from build123d import *

# Parameters (mm, degrees)
CROQUIS1_R              = 2.034348523
CROQUIS1_R_2            = 3
SALIENTE_EXTRUIR1_DEPTH = 3
SALIENTE_EXTRUIR2_DEPTH = 3
MATRIZC1_COUNT          = 8
MATRIZC1_ANGLE          = 128
CROQUIS4_R              = 1.53
CORTAR_EXTRUIR1_DEPTH   = 10


with BuildPart() as part:
    # Croquis1 → Saliente-Extruir1 (new body)
    with BuildSketch(Plane(origin=(0, 0, 0), x_dir=(1, 0, 0), z_dir=(0, 1, 0))):
        with BuildLine():
            Line((-5, -10.339498295), (-5, -30))
            ThreePointArc((-5, -30), (0, -35), (5, -30))
            Line((5, -30), (5, -10.339498295))
            ThreePointArc((5, -10.339498295), (0, 11.485), (-5, -10.339498295))
        make_face()
        with Locations((0, -30)):
            Circle(CROQUIS1_R, mode=Mode.SUBTRACT)
        Circle(CROQUIS1_R_2, mode=Mode.SUBTRACT)
    extrude(amount=SALIENTE_EXTRUIR1_DEPTH)

    # Croquis3 → Saliente-Extruir2 (add)
    with BuildSketch(Plane(origin=(0, 0, 0), x_dir=(1, 0, 0), z_dir=(0, 1, 0))):
        with BuildLine():
            Line((-1.1484375, 12.965487086), (-1.1484375, 11.427436996))
            ThreePointArc((-1.1484375, 11.427436996), (0, 11.485), (1.1484375, 11.427436996))
            Line((1.1484375, 11.427436996), (1.1484375, 12.965487086))
            Line((1.1484375, 12.965487086), (0.57421875, 14.536162804))
            ThreePointArc((0.57421875, 14.536162804), (0, 14.5475), (-0.57421875, 14.536162804))
            Line((-0.57421875, 14.536162804), (-1.1484375, 12.965487086))
        make_face()
    saliente_extruir2 = extrude(amount=SALIENTE_EXTRUIR2_DEPTH)

    # MatrizC1: Saliente-Extruir2 ×8 about axis
    matrizc1_axis = Axis((0, 0, 0), (0, 1, 0))
    for i in range(1, MATRIZC1_COUNT):
        add(saliente_extruir2.rotate(matrizc1_axis, i * MATRIZC1_ANGLE / (MATRIZC1_COUNT - 1)))

    # Croquis4 → Cortar-Extruir1 (cut)
    with BuildSketch(Plane.XZ):
        with Locations((0.448059245, -6.108589683)):
            Circle(CROQUIS4_R)
        with Locations((0, 6.125)):
            Circle(CROQUIS4_R)
    extrude(amount=-CORTAR_EXTRUIR1_DEPTH, mode=Mode.SUBTRACT)


solid = part.part
CAD build for the part. Positions are in the model's coordinates, mm. A direction names the side the tool comes from. Give positions to 0.01 mm unless a question says otherwise; leave off trailing zeros. Order: outer loops, then holes, each group sorted by start corner. A loop starts at its lowest first (then second) coordinate and runs counter-clockwise, first axis right, second up. Notation, with made-up numbers: (3, -7) - (17, -7) arc R22 cw to (17, 15) - close; hole circle Ø3 at (-31, 59). An arc over 180 degrees is marked (long way). Write each question's results on one line, items separated by ' | '.
1. Pin check, flat tips, straight feed: pin 1 (0.8 mm diameter, centred on y = 2, z = -12.5, fed in from +X); pin 2 (1 mm diameter, centred on x = 7.5, y = 2, fed in from +Z); pin 3 (0.8 mm diameter, centred on y = 1, z = -12, fed in from -X). Stop position of each tip, or through.
Calculated:
pin 1: stops at x = 1.15 | pin 2: stops at z = 9.11 | pin 3: stops at x = -8.78
2. Pull direction Z, two halves, no side cores. Call faces 1 (the face through (-13.42, 1.48, -3.17)), 2 (the face through (-7.49, 1.48, -11.55)), 3 (the face through (0, 1, 35)): released by +Z, released by -Z, zero draft, split by the parting line, or undercut.
Calculated:
face 1: undercut | face 2: released by -Z | face 3: released by +Z
3. 3-axis set-ups, long thin cutter, end or side, ignore diameter. For faces 4 (the face through (-13.74, 1.48, 1.2)), 5 (the face through (-6.78, 1.48, 9.27)), 6 (the face through (1.148, 1, -12)), 7 (the face through (-10.32, 1.48, -5.04)), 8 (the face through (-0.86, 1.48, -13.76)): which of +Z, -Z, +X, -X, +Y, -Y reach the whole face in a straight line?
Calculated:
face 4: -X, +Y, -Y | face 5: +Z, +Y, -Y | face 6: -Z, +X, +Y, -Y | face 7: +Y, -Y | face 8: -Z, +Y, -Y
4. Saw through at C-C on z = 22. List the corners of the cut face in (x, y), and give its area (3 significant figures).
Calculated:
outline: (-5, 0) - (5, 0) - (5, 3) - (-5, 3) - close | area: 30.0 mm2
5. Saw through at D-D on y = 1. Count the separate pieces of the cut face and the enclosed holes in it, and give its area (3 significant figures).
Calculated:
separate pieces: 1 | enclosed holes: 4 | area: 636 mm2
6. Saw through at A-A on z = 30.5. List the corners of the cut face in (x, y).
Calculated:
outline: (-4.97, 0) - (-1.97, 0) - (-1.97, 3) - (-4.97, 3) - close; (1.97, 0) - (4.97, 0) - (4.97, 3) - (1.97, 3) - close
7. Probe L1, parallel to Z at x = -12, y = 2.15; L2, parallel to Z at x = 0, y = 2.05 (1 decimal); L3, parallel to X at y = 1.55, z = 13.5. List the from-to ranges inside material, lowest first. Write a range as from..to.
Calculated:
L1: z = -8.22..-7.59, -4.84..-2.44, -0.85..1.45, 3.08..5.45 | L2: z = -14.5..-7.6, -4.6..-3, 3..4.6, 7.7..28, 32..35 | L3: x = -5..5
8. Saw through at B-B on x = 0. List the corners of the cut face in (y, z) (1 decimal).
Calculated:
outline: (0, -14.5) - (3, -14.5) - (3, -7.6) - (0, -7.6) - close; (0, -4.6) - (3, -4.6) - (3, -3) - (0, -3) - close; (0, 3) - (3, 3) - (3, 4.6) - (0, 4.6) - close; (0, 7.7) - (3, 7.7) - (3, 28) - (0, 28) - close; (0, 32) - (3, 32) - (3, 35) - (0, 35) - close
